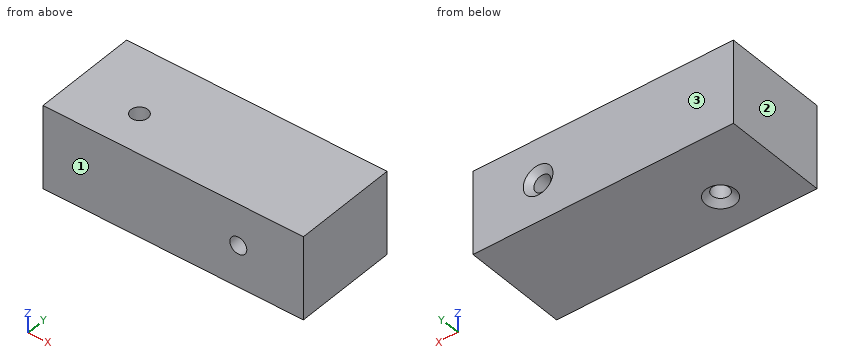
from build123d import *

# Parameters (mm, degrees)
SKETCH1_W                                         = 50
SKETCH1_H                                         = 20
BOSS_EXTRUDE1_DEPTH                               = 16
CSK_FOR_4_FLAT_HEAD_MACHINE_SCREW_100_D           = 3.2639
CSK_FOR_4_FLAT_HEAD_MACHINE_SCREW_100_DEPTH       = 16
CSK_FOR_4_FLAT_HEAD_MACHINE_SCREW_100_CSINK_D     = 5.715
CSK_FOR_4_FLAT_HEAD_MACHINE_SCREW_100_CSINK_ANGLE = 100
CSK_FOR_4_FLAT_HEAD_MACHINE_SCREW_2_D             = 3.2639
CSK_FOR_4_FLAT_HEAD_MACHINE_SCREW_2_DEPTH         = 20
CSK_FOR_4_FLAT_HEAD_MACHINE_SCREW_2_CSINK_D       = 5.715
CSK_FOR_4_FLAT_HEAD_MACHINE_SCREW_2_CSINK_ANGLE   = 100


with BuildPart() as part:
    # Sketch1 → Boss-Extrude1 (new body)
    with BuildSketch(Plane.XY):
        Rectangle(SKETCH1_W, SKETCH1_H)
    extrude(amount=-BOSS_EXTRUDE1_DEPTH)

    # CSK for _4 Flat Head Machine Screw _100
    with Locations(Plane(origin=(-12.5, -2.5, -16), x_dir=(-1, 0, 0), z_dir=(0, 0, -1))):
        with Locations((0, 0)):
            CounterSinkHole(CSK_FOR_4_FLAT_HEAD_MACHINE_SCREW_100_D / 2, CSK_FOR_4_FLAT_HEAD_MACHINE_SCREW_100_CSINK_D / 2, depth=CSK_FOR_4_FLAT_HEAD_MACHINE_SCREW_100_DEPTH, counter_sink_angle=CSK_FOR_4_FLAT_HEAD_MACHINE_SCREW_100_CSINK_ANGLE)

    # CSK for _4 Flat Head Machine Screw _ 2
    with Locations(Plane(origin=(0, 10, 0), x_dir=(1, 0, 0), z_dir=(0, 1, 0))):
        with Locations((12.5, 8)):
            CounterSinkHole(CSK_FOR_4_FLAT_HEAD_MACHINE_SCREW_2_D / 2, CSK_FOR_4_FLAT_HEAD_MACHINE_SCREW_2_CSINK_D / 2, depth=CSK_FOR_4_FLAT_HEAD_MACHINE_SCREW_2_DEPTH, counter_sink_angle=CSK_FOR_4_FLAT_HEAD_MACHINE_SCREW_2_CSINK_ANGLE)


solid = part.part
Geometry: final body of the model. Coordinates: model frame, mm. Face numbers are marked on the shaded views. Give positions to 0.01 mm unless a question says otherwise; leave off trailing zeros. Loops run counter-clockwise (first coordinate to the right, second up) from the corner with the lowest first, then second, coordinate; pieces in that order, holes last. Notation, with made-up numbers: (87, 8.25) -> (104, 8.25) arc R16 ccw to (104, 31.25) -> close; hole circle Ø10 at (63.5, 48). An arc over 180 degrees is marked (long way). Put each result on its own line as item: value.
1. Pull-direction query (Y, two-part tool) for the marked faces 1, 2 and 3; classes: released by +Y, released by -Y, zero draft, split by the parting line, or undercut.
Taken from the geometry:
face 1: released by -Y
face 2: zero draft
face 3: released by +Y
2. Cut plane C-C (y = -2.5). Return the cut outline in (x, z), plus the area to 3 significant figures.
Taken from the geometry:
outline: (-25, -16) -> (-15.36, -16) -> (-14.13, -14.97) -> (-14.13, 0) -> (-25, 0) -> close; (-10.87, -14.97) -> (-9.64, -16) -> (25, -16) -> (25, 0) -> (-10.87, 0) -> close; hole circle Ø3.26 at (12.5, -8)
area: 738 mm2
3. Ray query, line 1 along Z through (x, y) = (12.5, -3); line 2 along X through (y, z) = (-2.5, -6); line 3 along X through (y, z) = (3.75, -8). Return the intervals inside material, ascending. Write a range as [from, to].
Taken from the geometry:
line 1: z = [-16, -9.63], [-6.37, 0]
line 2: x = [-25, -14.13], [-10.87, 25]
line 3: x = [-25, 10.87], [14.13, 25]
4. Cut plane B-B (z = -8). Return the cut outline in (x, y).
Taken from the geometry:
outline: (-25, -10) -> (10.87, -10) -> (10.87, 8.97) -> (9.64, 10) -> (-25, 10) -> close; (14.13, -10) -> (25, -10) -> (25, 10) -> (15.36, 10) -> (14.13, 8.97) -> close; hole circle Ø3.26 at (-12.5, -2.5)
5. Pin query (flat end, axial travel): P1, Ø5, axis at x = 12.5, z = -8, coming from the +Y side. Return the tip coordinate at first contact, or that it passes through.
Taken from the geometry:
P1: stops at y = 9.7
6. Cut plane A-A (x = 12.5). Return the cut outline in (y, z).
Taken from the geometry:
outline: (-10, -16) -> (10, -16) -> (10, -10.86) -> (8.97, -9.63) -> (-10, -9.63) -> close; (-10, -6.37) -> (8.97, -6.37) -> (10, -5.14) -> (10, 0) -> (-10, 0) -> close
